Geometry: final body of the model. Coordinates: model frame, mm. Give positions to 0.01 mm unless a question says otherwise; leave off trailing zeros. Order: outer loops, then holes, each group sorted by start corner. A loop starts at its lowest first (then second) coordinate and runs counter-clockwise, first axis right, second up. Notation, with made-up numbers: (22.5, -7.5) -> (31.5, -7.5) arc R16 ccw to (31.5, 19.5) -> close; hole circle Ø9 at (84, -30.5). An arc over 180 degrees is marked (long way). One line per question, with ' | ' between items.
from build123d import *

# Parameters (mm, degrees)
SCHIZZO1_W                   = 15
SCHIZZO1_H                   = 23.8
SCHIZZO1_R                   = 1.25
ESTRUSIONE_ESTRUSIONE1_DEPTH = 2
RACCORDO1_R                  = 1
RACCORDO2_R                  = 1


with BuildPart() as part:
    # Schizzo1 → Estrusione-Estrusione1 (new body)
    with BuildSketch(Plane.XY):
        with Locations((-7.5, -11.9)):
            Rectangle(SCHIZZO1_W, SCHIZZO1_H)
        with Locations((-12, -5.1)):
            Circle(SCHIZZO1_R, mode=Mode.SUBTRACT)
        with Locations((-3.23, -21.8)):
            Circle(SCHIZZO1_R, mode=Mode.SUBTRACT)
    extrude(amount=ESTRUSIONE_ESTRUSIONE1_DEPTH)

    # Raccordo1
    raccordo1_edges = [part.edges().sort_by_distance(p)[0] for p in [
        (0, -23.8, 1),
        (-15, -23.8, 1),
        (-15, 0, 1),
        (0, 0, 1),
    ]]
    fillet(raccordo1_edges, radius=RACCORDO1_R)

    # Raccordo2
    # the kernel refuses this fillet: 1 mm, written as the material it takes off along each edge
    with BuildSketch(Plane(origin=(0, -22.8, 2), x_dir=(-1, 0, 0), z_dir=(0, 1, 0)), Plane(origin=(-15, -1, 2), x_dir=(1, 0, 0), z_dir=(0, -1, 0))) as raccordo2_piece_1:
        with BuildLine():
            CenterArc((RACCORDO2_R, -RACCORDO2_R), RACCORDO2_R, 90, 90)
            Line((0, -RACCORDO2_R), (0, 0))
            Line((0, 0), (RACCORDO2_R, 0))
        make_face()
    extrude(amount=21.8, mode=Mode.SUBTRACT)
    with BuildSketch(Plane(origin=(-14, -23.8, 2), x_dir=(0, 1, 0), z_dir=(1, 0, 0))) as raccordo2_piece_2:
        with BuildLine():
            CenterArc((RACCORDO2_R, -RACCORDO2_R), RACCORDO2_R, 90, 90)
            Line((0, -RACCORDO2_R), (0, 0))
            Line((0, 0), (RACCORDO2_R, 0))
        make_face()
    extrude(amount=13, mode=Mode.SUBTRACT)
    with BuildSketch(Plane(origin=(-1, 0, 2), x_dir=(0, 0, -1), z_dir=(-1, 0, 0))) as raccordo2_piece_3:
        with BuildLine():
            CenterArc((RACCORDO2_R, RACCORDO2_R), RACCORDO2_R, 180, 90)
            Line((0, RACCORDO2_R), (0, 0))
            Line((0, 0), (RACCORDO2_R, 0))
        make_face()
    extrude(amount=13, mode=Mode.SUBTRACT)
    with BuildSketch(Plane(origin=(-14, -22.8, 2), x_dir=(-1, 0, 0), z_dir=(0, 1, 0))) as raccordo2_piece_4:
        with BuildLine():
            CenterArc((1 - RACCORDO2_R, -RACCORDO2_R), RACCORDO2_R, 0, 90)
            Line((1, -RACCORDO2_R), (1, 0))
            Line((1, 0), (1 - RACCORDO2_R, 0))
        make_face()
    revolve(axis=Axis((-14, -22.8, 2), (0, 0, 1)), revolution_arc=90, mode=Mode.SUBTRACT)
    with BuildSketch(Plane(origin=(-14, -1, 2), x_dir=(0, 1, 0), z_dir=(1, 0, 0))) as raccordo2_piece_5:
        with BuildLine():
            CenterArc((1 - RACCORDO2_R, -RACCORDO2_R), RACCORDO2_R, 0, 90)
            Line((1 - RACCORDO2_R, 0), (1, 0))
            Line((1, 0), (1, -RACCORDO2_R))
        make_face()
    revolve(axis=Axis((-14, -1, 2), (0, 0, 1)), revolution_arc=90, mode=Mode.SUBTRACT)
    with BuildSketch(Plane(origin=(-1, -1, 2), x_dir=(0, 1, 0), z_dir=(-1, 0, 0))) as raccordo2_piece_6:
        with BuildLine():
            CenterArc((1 - RACCORDO2_R, RACCORDO2_R), RACCORDO2_R, 270, 90)
            Line((1 - RACCORDO2_R, 0), (1, 0))
            Line((1, 0), (1, RACCORDO2_R))
        make_face()
    revolve(axis=Axis((-1, -1, 2), (0, 0, -1)), revolution_arc=90, mode=Mode.SUBTRACT)
    with BuildSketch(Plane(origin=(-1, -22.8, 2), x_dir=(0, -1, 0), z_dir=(-1, 0, 0))) as raccordo2_piece_7:
        with BuildLine():
            CenterArc((1 - RACCORDO2_R, -RACCORDO2_R), RACCORDO2_R, 0, 90)
            Line((1, -RACCORDO2_R), (1, 0))
            Line((1, 0), (1 - RACCORDO2_R, 0))
        make_face()
    revolve(axis=Axis((-1, -22.8, 2), (0, 0, 1)), revolution_arc=90, mode=Mode.SUBTRACT)


solid = part.part
1) Section A-A on y = -21.8. Return loops of the section in (x, z).
Check result:
outline: (-15, 0) -> (-4.48, 0) -> (-4.48, 2) -> (-14, 2) arc R1 ccw to (-15, 1) -> close; (-1.98, 0) -> (0, 0) -> (0, 1) arc R1 ccw to (-1, 2) -> (-1.98, 2) -> close
2) Pull-direction query (Y, two-part tool) for faces 1 (the flat face through (-8, -12, 0)), 2 (the cylindrical face through (-12.921, -4.255, 0.986)), 3 (the cylindrical face through (-0.301, -23.515, 0.507)); classes: +Y half, -Y half, draft (parallel to the pull), parting line (faces both ways), or undercut.
Check result:
face 1: draft | face 2: undercut | face 3: -Y half
3) Section C-C on x = -12. Return loops of the section in (y, z).
Check result:
outline: (-23.8, 0) -> (-6.35, 0) -> (-6.35, 2) -> (-22.8, 2) arc R1 ccw to (-23.8, 1) -> close; (-3.85, 0) -> (0, 0) -> (0, 1) arc R1 ccw to (-1, 2) -> (-3.85, 2) -> close
4) Section D-D on z = 1.4. Return loops of the section in (x, y).
Check result:
outline: (-14.92, -22.8) arc R0.92 ccw to (-14, -23.72) -> (-1, -23.72) arc R0.92 ccw to (-0.08, -22.8) -> (-0.08, -1) arc R0.92 ccw to (-1, -0.08) -> (-14, -0.08) arc R0.92 ccw to (-14.92, -1) -> close; hole circle Ø2.5 at (-12, -5.1); hole circle Ø2.5 at (-3.23, -21.8)
5) Material intervals for probe 1 along X at (y, z) = (-21.8, 0.75); probe 2 along Y at (x, z) = (-12, 0.55); probe 3 along Y at (x, z) = (-3.75, 0.65), sorted ascending. Write a range as from..to.
Check result:
probe 1: x = -15..-4.48, -1.98..0 | probe 2: y = -23.8..-6.35, -3.85..0 | probe 3: y = -23.8..-22.94, -20.66..0
6) Section B-B on z = 0.25. Return loops of the section in (x, y), plus the area to 3 significant figures.
Check result:
outline: (-15, -22.8) arc R1 ccw to (-14, -23.8) -> (-1, -23.8) arc R1 ccw to (0, -22.8) -> (0, -1) arc R1 ccw to (-1, 0) -> (-14, 0) arc R1 ccw to (-15, -1) -> close; hole circle Ø2.5 at (-12, -5.1); hole circle Ø2.5 at (-3.23, -21.8) | area: 346 mm^2
